Geometry check sheet. Reference: drawing and pictorial views, mm from the part's lowest x, y, z. A direction names the side the tool comes from. Give positions to 0.01 mm unless a question says otherwise; leave off trailing zeros. Order: outer loops, then holes, each group sorted by start corner. A loop starts at its lowest first (then second) coordinate and runs counter-clockwise, first axis right, second up. Notation, with made-up numbers: (82.25, 10.5) -> (141.25, 10.5) arc R16 ccw to (141.25, 30.5) -> close; hole circle Ø6 at (66, -4). An arc over 180 degrees is marked (long way). Write each question's results on one line, items separated by ' | '.
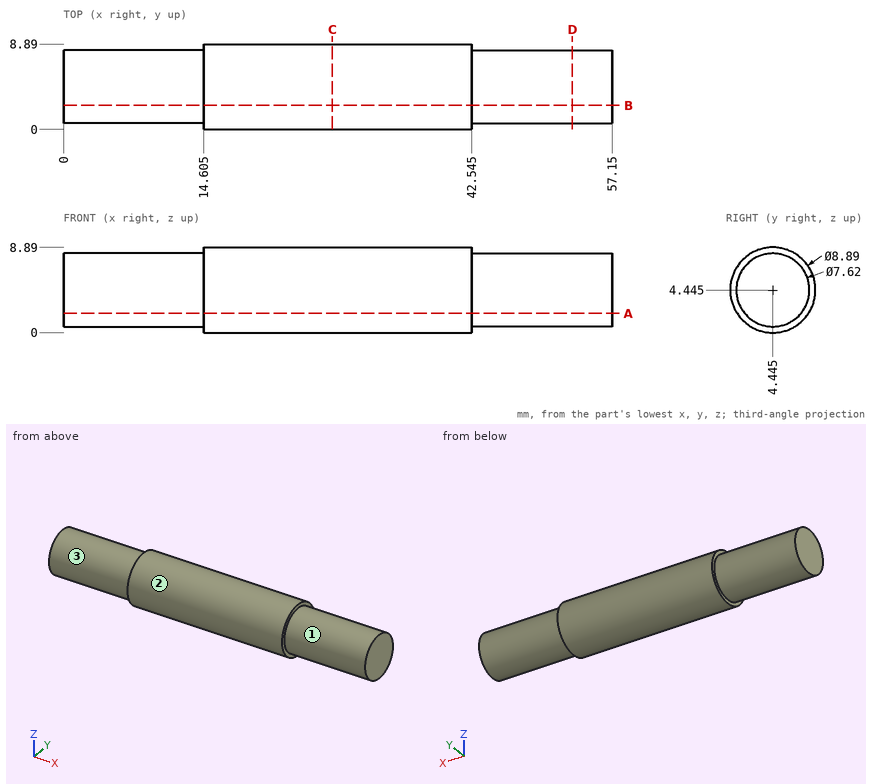
1. Section check A-A on z = 2. Record the cut outline in (x, y) (3 decimals).
Verdict:
outline: (0, 1.523) -> (14.605, 1.523) -> (14.605, 0.733) -> (42.545, 0.733) -> (42.545, 1.523) -> (57.15, 1.523) -> (57.15, 7.367) -> (42.545, 7.367) -> (42.545, 8.157) -> (14.605, 8.157) -> (14.605, 7.367) -> (0, 7.367) -> close
2. Section check D-D on x = 53. Record the cut outline in (y, z) (3 decimals).
Verdict:
outline: circle Ø7.62 at (4.445, 4.445)
3. Section check B-B on y = 2.5. Record the cut outline in (x, z) (3 decimals), then the cut area to 3 significant figures.
Verdict:
outline: (0, 1.169) -> (14.605, 1.169) -> (14.605, 0.448) -> (42.545, 0.448) -> (42.545, 1.169) -> (57.15, 1.169) -> (57.15, 7.721) -> (42.545, 7.721) -> (42.545, 8.442) -> (14.605, 8.442) -> (14.605, 7.721) -> (0, 7.721) -> close | area: 415 mm^2
4. Access from +Z, -Z, +X, -X, +Y, -Y to the whole of each face (thin tool, end or side, straight path). Record for the marked faces 1, 2 and 3.
Verdict:
face 1: +X | face 2: +X, -X | face 3: -X
5. Gauge pin test, flat ends, axial feed: pin 1 Ø2 at (x, z) = (45, 4.5) entering from +Y (3 decimals); pin 2 Ø2 at (x, z) = (27.5, 3) entering from -Y; pin 3 Ø4 at (x, z) = (21, 1) entering from +Y. Record the tip position at first contact, or that the pin passes through.
Verdict:
pin 1: stops at y = 8.255 | pin 2: stops at y = 0.02 | pin 3: stops at y = 8.65
6. Section check C-C on x = 28. Record the cut outline in (y, z) (3 decimals).
Verdict:
outline: circle Ø8.89 at (4.445, 4.445)
7. Material ranges on probe 1 along X at (y, z) = (8.25, 5.25) (3 decimals); probe 2 along Y at (x, z) = (41.5, 4.75); probe 3 along Y at (x, z) = (7, 4.25), recorded low to high. Write a range as from..to.
Verdict:
probe 1: x = 14.605..42.545 | probe 2: y = 0.01..8.88 | probe 3: y = 0.64..8.25
